The figure shows three views and two pictorial views of one solid part (mm, origin at its lowest corner). Answer the questions. A direction names the side the tool comes from. Coordinates: 2 decimals unless noted, no trailing zeros. Loops run counter-clockwise (first coordinate to the right, second up) from the corner with the lowest first, then second, coordinate; pieces in that order, holes last. Notation, with made-up numbers: M 11.25,57.5 L 64.25,57.5 A20 cw 64.25,75.5 Z; hole C 36.25,-15.5 d3. An arc over 180 degrees is marked long. Answer as a JSON object with one key per item and string values. Group by question number.
1. For the marked faces 1, 2 and 3, determine the directions among +Z, -Z, +X, -X, +Y, -Y from which every point of the face is accessible in a straight line to the end or side of a thin tool.
2. Given pin 1 (3 mm diameter, centred on x = 21.5, y = 2, fed in from +Z); pin 2 (3 mm diameter, centred on y = 12.5, z = 2.5, fed in from +X); pin 3 (2 mm diameter, centred on y = 12, z = 2.5, fed in from -X); pin 4 (3 mm diameter, centred on x = 9, y = 2, fed in from -Z), each flat-ended and moving along its own axis, determine where each tip first touches the part or whether it passes through.
3. Straight lines are drawn through the part: L1, parallel to Y at x = 21.5, z = 5.65; L2, parallel to Z at x = 5.75, y = 6; L3, parallel to X at y = 9.25, z = 1.1. For each, find the intervals that lie inside material, in ascending order.
4. A cutting plane is placed at B-B on x = 21.5. Give the vertices of the cut face in (y, z).
5. A cutting plane is placed at A-A on y = 2. Give the vertices of the cut face in (x, z).
6. A cutting plane is placed at C-C on y = 12.5. Give the vertices of the cut face in (x, z), and give its area (3 significant figures).
7. A cutting plane is placed at D-D on x = 11.25. Give the vertices of the cut face in (y, z), and give its area (3 significant figures).
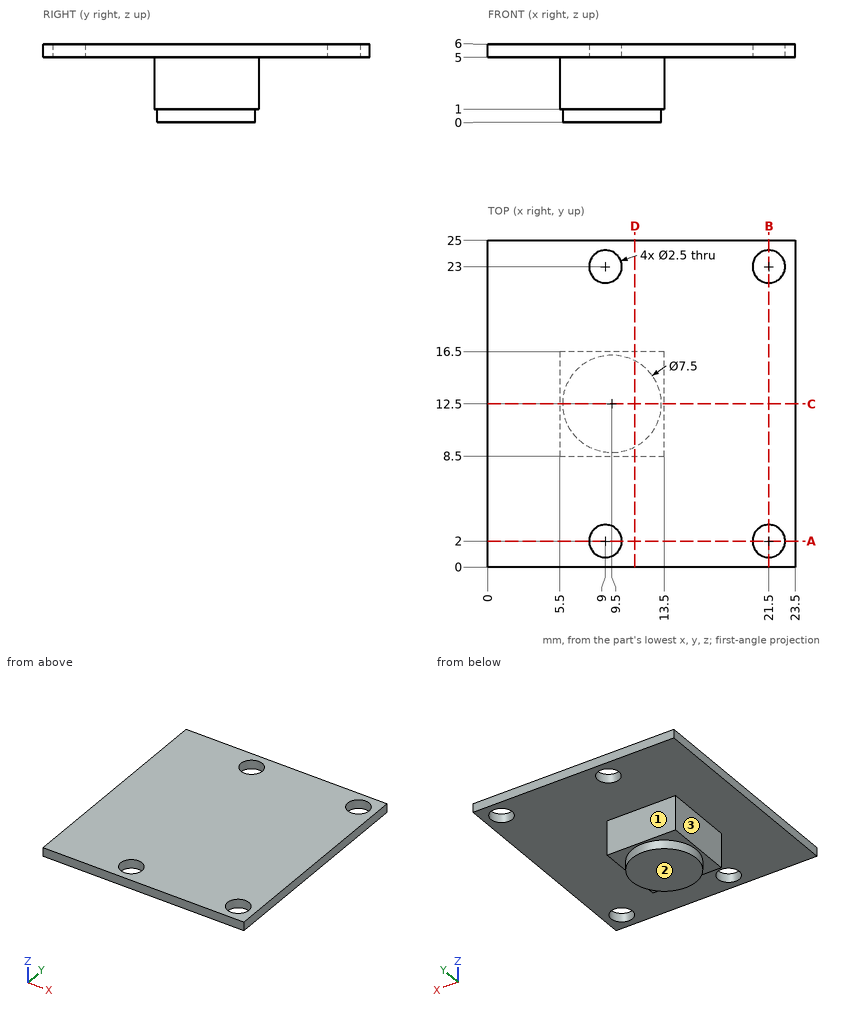
From the geometry:
{
 "1": {"face 1": "-Z, +X, -X, +Y", "face 2": "-Z, +X, -X, +Y, -Y", "face 3": "-Z, -X, +Y, -Y"},
 "2": {"pin 1": "stops at z = 6", "pin 2": "stops at x = 13.5", "pin 3": "stops at x = 5.5", "pin 4": "stops at z = 5"},
 "3": {"L1": "y = 0 to 0.75, 3.25 to 21.75, 24.25 to 25", "L2": "z = 5 to 6", "L3": "x = 5.5 to 13.5"},
 "4": {"outline": "M 0,5 L 0.75,5 L 0.75,6 L 0,6 Z; M 3.25,5 L 21.75,5 L 21.75,6 L 3.25,6 Z; M 24.25,5 L 25,5 L 25,6 L 24.25,6 Z"},
 "5": {"outline": "M 0,5 L 7.75,5 L 7.75,6 L 0,6 Z; M 10.25,5 L 20.25,5 L 20.25,6 L 10.25,6 Z; M 22.75,5 L 23.5,5 L 23.5,6 L 22.75,6 Z"},
 "6": {"outline": "M 0,5 L 5.5,5 L 5.5,1 L 5.75,1 L 5.75,0 L 13.25,0 L 13.25,1 L 13.5,1 L 13.5,5 L 23.5,5 L 23.5,6 L 0,6 Z", "area": "63.0 mm²"},
 "7": {"outline": "M 0,5 L 8.5,5 L 8.5,1 L 9.18,1 L 9.18,0 L 15.82,0 L 15.82,1 L 16.5,1 L 16.5,5 L 25,5 L 25,6 L 0,6 Z", "area": "63.6 mm²"}
}
